Answer from the drawing. Dimensions are ordinates in mm from the lowest x, y and z of the part. Give positions to 0.01 mm unless a question says otherwise; leave off trailing zeros. Loops run counter-clockwise (first coordinate to the right, second up) from the corner with the lowest first, then second, coordinate; pieces in that order, holes last. Notation, with made-up numbers: (18, -5) -> (26, -5) arc R27 ccw to (26, 34) -> close; hole circle Ø7 at (41.25, -30.5). An arc over 180 degrees is marked (long way). Answer as CSV lines item,"result". Start each with the question number.
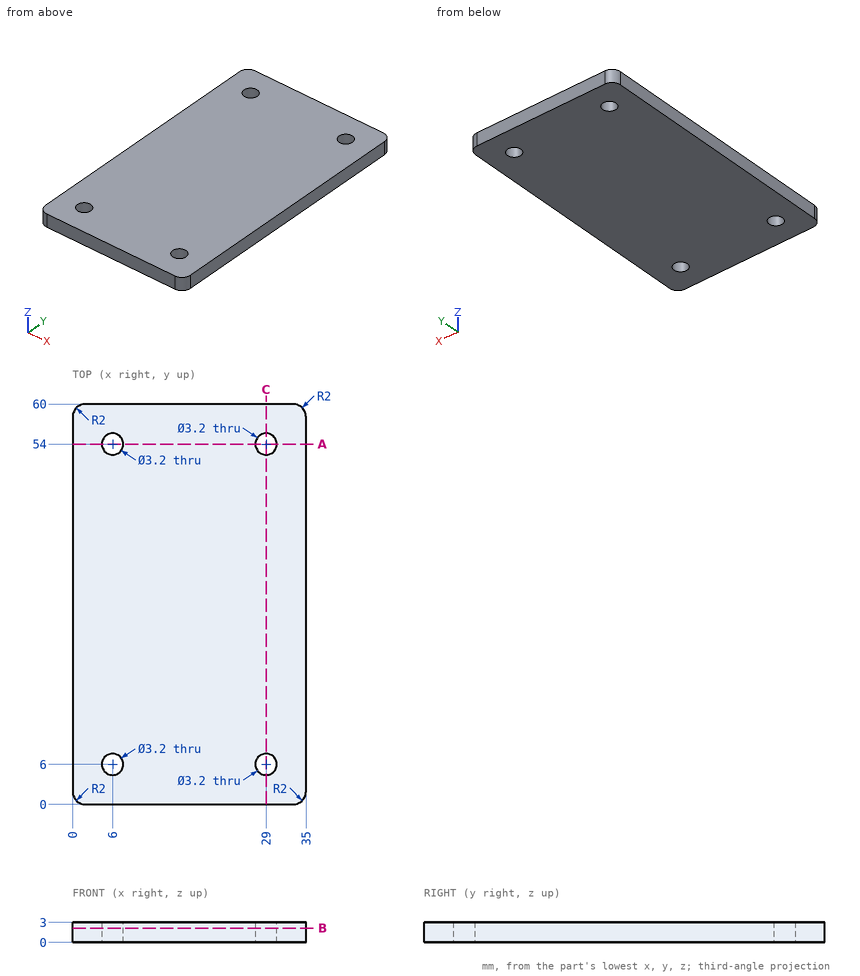
(1) Find section B-B on z = 2.15. Write down the section's boundary in (x, y), then the cut area to 3 significant figures.
(2) This flat-tipped pin is pushed along its axis until it touches: P1, Ø2, axis at x = 22.5, y = 50, coming from the -Z side. Where does it stop, or does it pass through?
(3) Find the intervals of material crossed by line 1 along Y through (x, z) = (6, 1.15); line 2 along X through (y, z) = (5, 2.35); line 3 along Y through (x, z) = (29.5, 2.8), in increasing order. Write a range as from..to.
(4) Find section A-A on y = 54. Write down the section's boundary in (x, z).
(5) Find section C-C on x = 29. Write down the section's boundary in (y, z).
Answer block:
1,outline,"(0, 2) arc R2 ccw to (2, 0) -> (33, 0) arc R2 ccw to (35, 2) -> (35, 58) arc R2 ccw to (33, 60) -> (2, 60) arc R2 ccw to (0, 58) -> close; hole circle Ø3.2 at (6, 6); hole circle Ø3.2 at (6, 54); hole circle Ø3.2 at (29, 6); hole circle Ø3.2 at (29, 54)"
1,area,"2,060 mm2"
2,P1,"stops at z = 0"
3,line 1,"y = 0..4.4, 7.6..52.4, 55.6..60"
3,line 2,"x = 0..4.75, 7.25..27.75, 30.25..35"
3,line 3,"y = 0..4.48, 7.52..52.48, 55.52..60"
4,outline,"(0, 0) -> (4.4, 0) -> (4.4, 3) -> (0, 3) -> close; (7.6, 0) -> (27.4, 0) -> (27.4, 3) -> (7.6, 3) -> close; (30.6, 0) -> (35, 0) -> (35, 3) -> (30.6, 3) -> close"
5,outline,"(0, 0) -> (4.4, 0) -> (4.4, 3) -> (0, 3) -> close; (7.6, 0) -> (52.4, 0) -> (52.4, 3) -> (7.6, 3) -> close; (55.6, 0) -> (60, 0) -> (60, 3) -> (55.6, 3) -> close"
